Read the model definition and answer for the solid it produces. Units are mm, in the model's axes. Face numbers are marked on the shaded views. A direction names the side the tool comes from. Give positions to 0.01 mm unless a question says otherwise; leave off trailing zeros. Order: outer loops, then holes, each group sorted by start corner. A loop starts at its lowest first (then second) coordinate and runs counter-clockwise, first axis right, second up. Notation, with made-up numbers: (-31.75, 48.5) - (6.25, 48.5) arc R21 cw to (6.25, 79.5) - close; hole circle Ø4 at (-35.75, 14.25). An arc over 180 degrees is marked (long way). Write item = value, one per line.
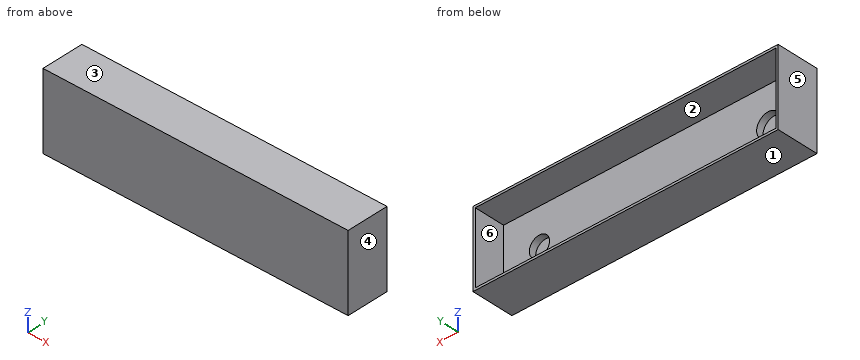
```python
from build123d import *

# Parameters (mm, degrees)
SKETCH1_W           = 400
SKETCH1_H           = 100
BOSS_EXTRUDE1_DEPTH = 15
SKETCH2_R           = 15.25
SKETCH2_R_2         = 13.25
CUT_EXTRUDE1_DEPTH  = 9
SKETCH3_W           = 400
SKETCH3_H           = 100
SKETCH3_W_2         = 394
SKETCH3_H_2         = 94
BOSS_EXTRUDE2_DEPTH = 40


with BuildPart() as part:
    # Sketch1 → Boss-Extrude1 (new body)
    with BuildSketch(Plane(origin=(0, 0, 0), x_dir=(1, 0, 0), z_dir=(0, 1, 0))):
        Rectangle(SKETCH1_W, SKETCH1_H)
    extrude(amount=BOSS_EXTRUDE1_DEPTH)

    # Sketch2 → Cut-Extrude1 (cut)
    with BuildSketch(Plane(origin=(0, 15, 0), x_dir=(1, 0, 0), z_dir=(0, 1, 0))):
        with Locations(Location((-150, 0, 0), (0, 0, 270))):
            Circle(SKETCH2_R)
        with Locations(Location((150, 0, 0), (0, 0, 270))):
            Circle(SKETCH2_R_2)
    extrude(amount=-CUT_EXTRUDE1_DEPTH, mode=Mode.SUBTRACT)

    # Sketch3 → Boss-Extrude2 (add)
    with BuildSketch(Plane(origin=(0, 15, 0), x_dir=(1, 0, 0), z_dir=(0, 1, 0))):
        Rectangle(SKETCH3_W, SKETCH3_H)
        Rectangle(SKETCH3_W_2, SKETCH3_H_2, mode=Mode.SUBTRACT)
    extrude(amount=BOSS_EXTRUDE2_DEPTH)


solid = part.part
```
1. Determine the mould class of the marked faces 1, 2, 3 and 4 for opening direction Z: +Z half, -Z half, draft (parallel to the pull), parting line (faces both ways), or undercut.
Recorded:
face_1 = -Z half
face_2 = undercut
face_3 = +Z half
face_4 = draft
2. Section D-D (x = 150) is taken. Determine the outline of the cut face in (y, z), and give its area (3 significant figures).
Recorded:
outline = (0, -50) - (55, -50) - (55, -47) - (15, -47) - (15, -13.25) - (6, -13.25) - (6, 13.25) - (15, 13.25) - (15, 47) - (55, 47) - (55, 50) - (0, 50) - close
area = 1,500 mm^2
3. Section C-C (z = -30) is taken. Determine the outline of the cut face in (x, y), and give its area (3 significant figures).
Recorded:
outline = (-200, 0) - (200, 0) - (200, 55) - (197, 55) - (197, 15) - (-197, 15) - (-197, 55) - (-200, 55) - close
area = 6,240 mm^2
4. Section A-A (x = 63.5) is taken. Determine the outline of the cut face in (y, z), and give its area (3 significant figures).
Recorded:
outline = (0, -50) - (55, -50) - (55, -47) - (15, -47) - (15, 47) - (55, 47) - (55, 50) - (0, 50) - close
area = 1,740 mm^2
5. Section B-B (y = 19) is taken. Determine the outline of the cut face in (x, z), and give its area (3 significant figures).
Recorded:
outline = (-200, -50) - (200, -50) - (200, 50) - (-200, 50) - close; hole (-197, -47) - (197, -47) - (197, 47) - (-197, 47) - close
area = 2,960 mm^2
6. Flat-ended cylindrical pins translate along their axes: pin 1 (21 mm diameter, centred on x = 150, z = 0, fed in from +Y); pin 2 (2 mm diameter, centred on x = -3.5, z = -10.5, fed in from +Y). Find the tip coordinate at first contact, or state that the pin passes through.
Recorded:
pin_1 = 6
pin_2 = 15
7. Straight lines are drawn through the part: L1, parallel to X at y = 8.5, z = 0; L2, parallel to Z at x = 69.5, y = 32.5; L3, parallel to X at y = 44, z = -26. For each, find the intervals that lie inside material, in ascending order. Write a range as [from, to].
Recorded:
L1 = [-200, -165.25], [-134.75, 136.75], [163.25, 200]
L2 = [-50, -47], [47, 50]
L3 = [-200, -197], [197, 200]
8. For the marked faces 5 and 6, determine the directions among +Z, -Z, +X, -X, +Y, -Y from which every point of the face is accessible in a straight line to the end or side of a thin tool.
Recorded:
face_5 = +Z, -Z, -X, +Y, -Y
face_6 = +Y
